Input: part model. Units: mm. Frame: model coordinates. Coordinates: 2 decimals unless noted, no trailing zeros. Loops run counter-clockwise (first coordinate to the right, second up) from the corner with the lowest first, then second, coordinate; pieces in that order, holes last.
(1) Section D-D, the plane y = 18. Return loops of the section in (x, z), then the cut area to 3 significant figures.
(2) Section B-B, the plane z = 1.05. Return loops of the section in (x, y).
(3) Contact query for a flat-ended pin moving along its axis: P1, Ø0.8, axis at x = 110.5, z = 0.5, coming from the -Y side. Output: stop coordinate, or through.
(4) Line query: L1, parallel to X at y = 2.5, z = 1.05; L2, parallel to X at y = 12.75, z = 0.1; L3, parallel to Y at x = 195.5, z = 0.35. Output: solid intervals per line, ascending.
(5) Section C-C, the plane x = 50. Return loops of the section in (y, z).
(6) Section A-A, the plane y = 6. Return loops of the section in (x, z).
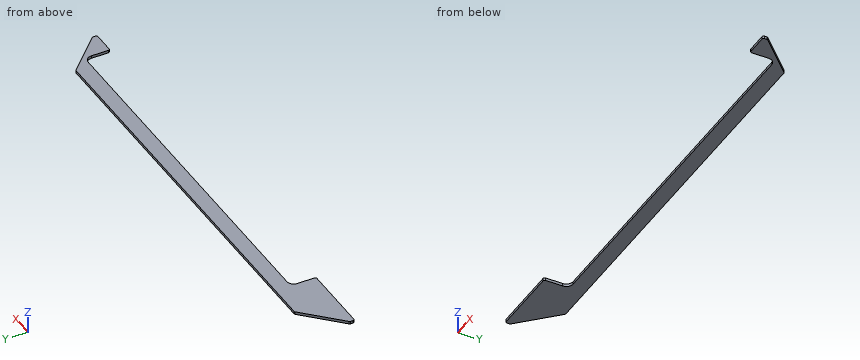
```python
from build123d import *

# Parameters (mm, degrees)
BOSS_EXTRUDE1_DEPTH = 1.6
FILLET1_R           = 1


with BuildPart() as part:
    # Sketch1 → Boss-Extrude1 (new body)
    with BuildSketch(Plane.XY):
        with BuildLine():
            Line((21.213203436, 24), (0, 2.786796564))
            Line((0, 2.786796564), (0, 0))
            Line((0, 0), (42, 0))
            Line((42, 0), (42, 11))
            ThreePointArc((42, 11), (43.171572875, 13.828427125), (46, 15))
            Line((46, 15), (262, 15))
            ThreePointArc((262, 15), (264.828427125, 13.828427125), (266, 11))
            Line((266, 11), (266, 0))
            Line((266, 0), (280, 0))
            Line((280, 0), (280, 2.786796564))
            Line((280, 2.786796564), (258.786796564, 24))
            Line((258.786796564, 24), (21.213203436, 24))
        make_face()
    extrude(amount=BOSS_EXTRUDE1_DEPTH)

    # Fillet1
    fillet1_edges = [part.edges().sort_by_distance(p)[0] for p in [
        (42, 0, 0.8),
        (0, 0, 0.8),
        (0, 2.786796564, 0.8),
        (21.213203436, 24, 0.8),
        (258.786796564, 24, 0.8),
        (280, 2.786796564, 0.8),
        (280, 0, 0.8),
        (266, 0, 0.8),
    ]]
    fillet(fillet1_edges, radius=FILLET1_R)


solid = part.part
```
Report:
1. outline: (15.21, 0) - (264.79, 0) - (264.79, 1.6) - (15.21, 1.6) - close
1. area: 399 mm2
2. outline: (0, 1) arc R1 ccw to (1, 0) - (41, 0) arc R1 ccw to (42, 1) - (42, 11) arc R4 cw to (46, 15) - (262, 15) arc R4 cw to (266, 11) - (266, 1) arc R1 ccw to (267, 0) - (279, 0) arc R1 ccw to (280, 1) - (280, 2.37) arc R1 ccw to (279.71, 3.08) - (259.08, 23.71) arc R1 ccw to (258.37, 24) - (21.63, 24) arc R1 ccw to (20.92, 23.71) - (0.29, 3.08) arc R1 ccw to (0, 2.37) - close
3. P1: stops at y = 15
4. L1: x = 0.01 to 42, 266 to 279.99
4. L2: x = 9.96 to 42.4, 265.6 to 270.04
4. L3: y = 15 to 24
5. outline: (15, 0) - (24, 0) - (24, 1.6) - (15, 1.6) - close
6. outline: (3.21, 0) - (42, 0) - (42, 1.6) - (3.21, 1.6) - close; (266, 0) - (276.79, 0) - (276.79, 1.6) - (266, 1.6) - close
